Geometry: see drawing. Coordinates: mm, zero at the bounding-box minimum. Coordinates: 2 decimals unless noted, no trailing zeros. Loops run counter-clockwise (first coordinate to the right, second up) from the corner with the lowest first, then second, coordinate; pieces in that order, holes last. Notation, with made-up numbers: (-24.5, -1.5) - (25.5, -1.5) arc R36 ccw to (25.5, 32.5) - close; hole circle Ø3 at (-8, 39.5). An arc over 180 degrees is marked (long way). Use one line per item in the form item = value.
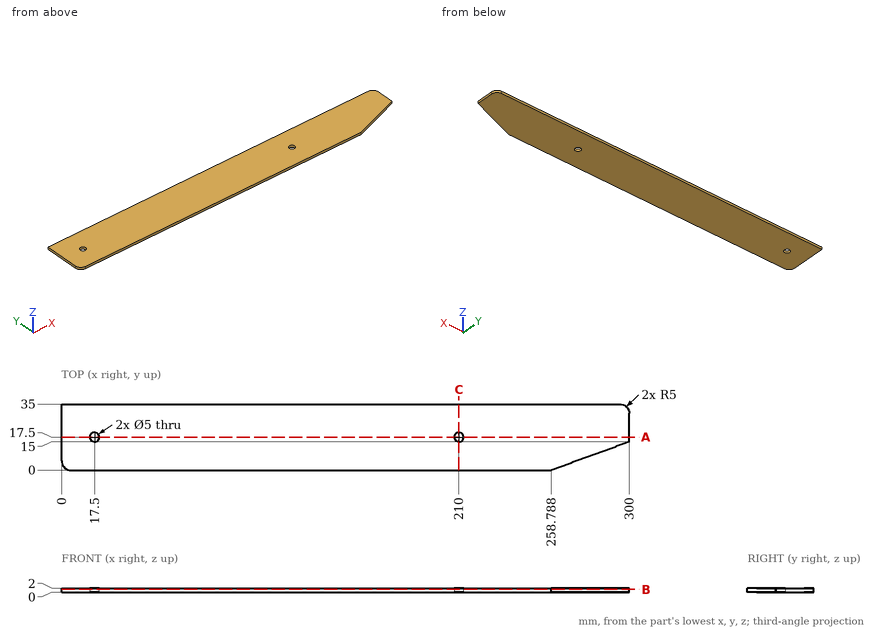
Q1. First-contact query: P1, Ø4, axis at x = 210, y = 17.5, coming from the +Z side. Flat tip, straight axial feed; report the tip coordinate or a pass-through.
Check values:
P1 = through
Q2. Ray query, line 1 along Y through (x, z) = (17.5, 0.95); line 2 along X through (y, z) = (33.5, 1.5). Return the intervals inside material, ascending. Write a range as [from, to].
Check values:
line_1 = [0, 15], [20, 35]
line_2 = [0, 298.57]
Q3. Cut plane B-B, the plane z = 1.35. Return loops of the section in (x, y).
Check values:
outline = (0, 5) arc R5 ccw to (5, 0) - (258.79, 0) - (300, 15) - (300, 30) arc R5 ccw to (295, 35) - (0, 35) - close; hole circle Ø5 at (17.5, 17.5); hole circle Ø5 at (210, 17.5)
Q4. Cut plane A-A, the plane y = 17.5. Return loops of the section in (x, z), then the cut area to 3 significant figures.
Check values:
outline = (0, 0) - (15, 0) - (15, 2) - (0, 2) - close; (20, 0) - (207.5, 0) - (207.5, 2) - (20, 2) - close; (212.5, 0) - (300, 0) - (300, 2) - (212.5, 2) - close
area = 580 mm²
Q5. Cut plane C-C, the plane x = 210. Return loops of the section in (y, z).
Check values:
outline = (0, 0) - (15, 0) - (15, 2) - (0, 2) - close; (20, 0) - (35, 0) - (35, 2) - (20, 2) - close
